Verification items for the finished model (mm, model axes). Face numbers are marked on the shaded views. A direction names the side the tool comes from. Round coordinates to 2 decimals unless told otherwise and drop trailing zeros. Order: outer loops, then holes, each group sorted by start corner. A loop starts at its lowest first (then second) coordinate and runs counter-clockwise, first axis right, second up. Notation, with made-up numbers: (48, 37.25) -> (67, 37.25) arc R35 ccw to (67, 75.25) -> close; hole circle Ø3 at (14.25, -4). An arc over 180 degrees is marked (long way). Return JSON: item names as keys, results as strings. Group by question number.
Item 1: Depth check by flat-ended pin: pin 1 Ø3 at (x, z) = (-11, 10) entering from -Y; pin 2 Ø4.5 at (y, z) = (-4, 3.5) entering from +X. Enter the tip coordinate at first touch or a pass-through.
Item 2: Draft check along X on the marked faces 3, 4 and 5. Enter one of: pulls with the +X half, pulls with the -X half, needs draft (parallel to the pull), parting line crosses it, or undercut.
Item 3: Sectioned sample at A-A on y = -13.25. Record the cut outline in (x, z).
Item 4: Sectioned sample at D-D on z = -1. Record the cut outline in (x, y), plus the area to 3 significant figures.
Item 5: Access from +Z, -Z, +X, -X, +Y, -Y to the whole of each face (thin tool, end or side, straight path). Record for the marked faces 1 and 2.
Item 6: Sectioned sample at B-B on z = -30.5. Record the cut outline in (x, y).
Item 7: Scan lines: probe 1 along X at (y, z) = (-2.25, -31); probe 2 along Y at (x, z) = (30, 31.5); probe 3 along X at (y, z) = (-4, 11). Record each from-to range of solid material in increasing order. Write a range as from..to.
Item 8: Sectioned sample at C-C on x = 54. Record the cut outline in (y, z), plus the area to 3 significant figures.
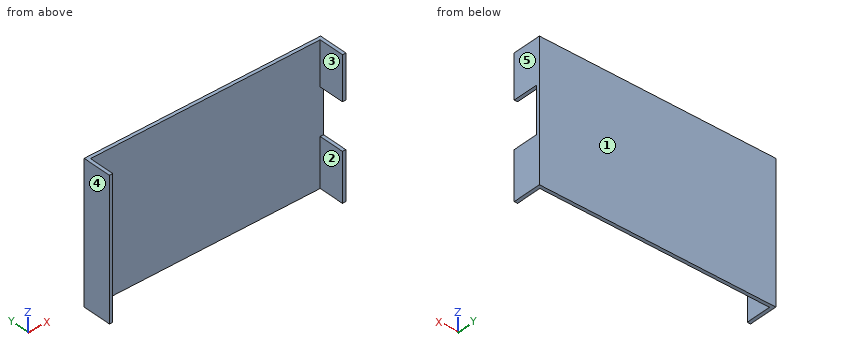
```python
from build123d import *

# Parameters (mm, degrees)
EXTRUDE_1_DEPTH     = 2
SKETCH_2_W          = 2
SKETCH_2_H          = 82
EXTRUDE_2_DEPTH     = 15
CUT_EXTRUDE_2_DEPTH = 20


with BuildPart() as part:
    # 草图1 → 凸台-拉伸1 (new body)
    with BuildSketch(Plane(origin=(0, 0, 0), x_dir=(1, 0, 0), z_dir=(0, 1, 0))):
        Polygon((0, -41), (70, -41), (70, -6.017578489), (70, 41), (0, 41), (-70, 41), (-70, 0), (-70, -41), align=None)
    extrude(amount=EXTRUDE_1_DEPTH)

    # 草图2 → 凸台-拉伸2 (add)
    with BuildSketch(Plane.XZ):
        with Locations((-69, 0)):
            Rectangle(SKETCH_2_W, SKETCH_2_H)
        with Locations((69, 0)):
            Rectangle(SKETCH_2_W, SKETCH_2_H)
    extrude(amount=EXTRUDE_2_DEPTH)

    # 草图4 → 切除-拉伸2 (cut)
    with BuildSketch(Plane(origin=(70, 0, 0), x_dir=(0, 0, -1), z_dir=(1, 0, 0))):
        Polygon((0, 0), (-14.99, 0), (-14.99, -15), (12.32, -15), (12.32, 0), align=None)
    extrude(amount=-CUT_EXTRUDE_2_DEPTH, mode=Mode.SUBTRACT)


solid = part.part
```
Recorded:
{
 "1": {"pin 1": "y = 0", "pin 2": "x = -68"},
 "2": {"face 3": "undercut", "face 4": "pulls with the -X half", "face 5": "pulls with the +X half"},
 "3": {"outline": "(-70, -41) -> (-68, -41) -> (-68, 41) -> (-70, 41) -> close; (68, -41) -> (70, -41) -> (70, -12.32) -> (68, -12.32) -> close; (68, 14.99) -> (70, 14.99) -> (70, 41) -> (68, 41) -> close"},
 "4": {"outline": "(-70, -15) -> (-68, -15) -> (-68, 0) -> (70, 0) -> (70, 2) -> (-70, 2) -> close", "area": "310 mm²"},
 "5": {"face 1": "+Z, -Z, +X, -X, +Y", "face 2": "+Z, -Z, -Y"},
 "6": {"outline": "(-70, -15) -> (-68, -15) -> (-68, 0) -> (68, 0) -> (68, -15) -> (70, -15) -> (70, 2) -> (-70, 2) -> close"},
 "7": {"probe 1": "-70..-68, 68..70", "probe 2": "0..2", "probe 3": "-70..-68"},
 "8": {"outline": "(0, -41) -> (2, -41) -> (2, 41) -> (0, 41) -> close", "area": "164 mm²"}
}
